CAD build for the part. Positions are in the model's coordinates, mm. Face numbers are marked on the shaded views. A direction names the side the tool comes from. Coordinates: 2 decimals unless noted, no trailing zeros. Loops run counter-clockwise (first coordinate to the right, second up) from the corner with the lowest first, then second, coordinate; pieces in that order, holes last. Notation, with made-up numbers: (-40, 86.25) -> (0, 86.25) arc R13 cw to (0, 97.25) -> close; hole circle Ø4 at (-23, 4). An arc over 180 degrees is marked (long way). Write each question's results on one line, items separated by ' | '.
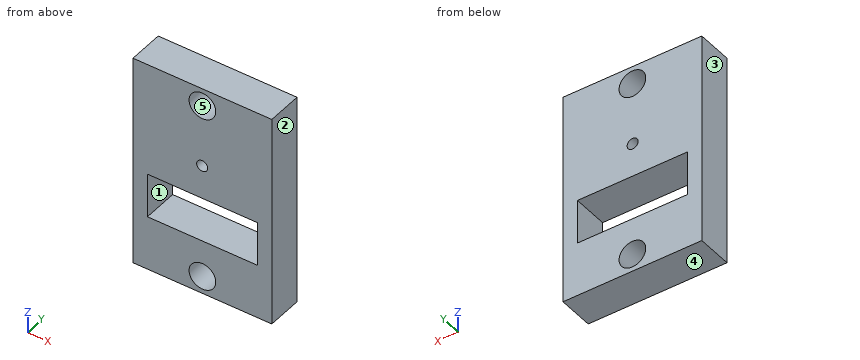
```python
from build123d import *

# Parameters (mm, degrees)
SKETCH1_W           = 78
SKETCH1_H           = 120
BOSS_EXTRUDE1_DEPTH = 10
CUT_EXTRUDE1_REACH  = 102.419
SKETCH2_W           = 61.75
SKETCH2_H           = 25
CUT_EXTRUDE2_REACH  = 102.419
SKETCH3_R           = 7.5
CUT_EXTRUDE3_REACH  = 102.419
SKETCH5_R           = 3.1


with BuildPart() as part:
    # Sketch1 → Boss-Extrude1 (new, symmetric)
    with BuildSketch(Plane(origin=(0, 0, 0), x_dir=(1, 0, 0), z_dir=(0, 1, 0))):
        with Locations((-39, 0)):
            Rectangle(SKETCH1_W, SKETCH1_H)
    extrude(amount=BOSS_EXTRUDE1_DEPTH, both=True)

    # Sketch2 → Cut-Extrude1 (cut, up to next)
    with BuildSketch(Plane(origin=(0, 10, 0), x_dir=(1, 0, 0), z_dir=(0, 1, 0)), mode=Mode.PRIVATE) as cut_extrude1_sk1:
        with Locations((-39, 16.78)):
            Rectangle(SKETCH2_W, SKETCH2_H)
    cut_extrude1_tool1 = extrude(cut_extrude1_sk1.sketch, amount=-CUT_EXTRUDE1_REACH, mode=Mode.PRIVATE) & part.part
    add(cut_extrude1_tool1.solids().sort_by_distance((-39, 10, -16.78))[0], mode=Mode.SUBTRACT)

    # Sketch3 → Cut-Extrude2 (cut, up to next)
    with BuildSketch(Plane(origin=(0, 10, 0), x_dir=(1, 0, 0), z_dir=(0, 1, 0)), mode=Mode.PRIVATE) as cut_extrude2_sk1:
        with Locations(Location((-39, 50, 0), (0, 0, 270))):
            Circle(SKETCH3_R)
    cut_extrude2_tool1 = extrude(cut_extrude2_sk1.sketch, amount=-CUT_EXTRUDE2_REACH, mode=Mode.PRIVATE) & part.part
    # Sketch3 → Cut-Extrude2 (cut, up to next)
    with BuildSketch(Plane(origin=(0, 10, 0), x_dir=(1, 0, 0), z_dir=(0, 1, 0)), mode=Mode.PRIVATE) as cut_extrude2_sk2:
        with Locations(Location((-39, -50, 0), (0, 0, 270))):
            Circle(SKETCH3_R)
    cut_extrude2_tool2 = extrude(cut_extrude2_sk2.sketch, amount=-CUT_EXTRUDE2_REACH, mode=Mode.PRIVATE) & part.part
    add(cut_extrude2_tool1.solids().sort_by_distance((-39, 10, -50))[0], mode=Mode.SUBTRACT)
    add(cut_extrude2_tool2.solids().sort_by_distance((-39, 10, 50))[0], mode=Mode.SUBTRACT)

    # Sketch5 → Cut-Extrude3 (cut, up to next)
    with BuildSketch(Plane(origin=(0, 10, 0), x_dir=(1, 0, 0), z_dir=(0, 1, 0)), mode=Mode.PRIVATE) as cut_extrude3_sk1:
        with Locations(Location((-39.125, -14.72, 0), (0, 0, 270))):
            Circle(SKETCH5_R)
    cut_extrude3_tool1 = extrude(cut_extrude3_sk1.sketch, amount=-CUT_EXTRUDE3_REACH, mode=Mode.PRIVATE) & part.part
    add(cut_extrude3_tool1.solids().sort_by_distance((-39.125, 10, 14.72))[0], mode=Mode.SUBTRACT)


solid = part.part
```
Q1. Drop a flat-ended pin along its axis: pin 1 (12 mm diameter, centred on x = -39, z = -50, fed in from +Y) (1 decimal). Give the stop position or say it passes through.
Results are:
pin 1: through
Q2. Which spindle directions (+Z, -Z, +X, -X, +Y, -Y) get a long thin tool onto all of the face, cutting with end or side? Do the marked faces 1 and 2. Say none if no direction does.
Results are:
face 1: +Y, -Y | face 2: +Z, -Z, +X, +Y, -Y
Q3. Cut at C-C on y = -2.5. Write the cut outline in (x, z) (3 decimals), and give its area (3 significant figures).
Results are:
outline: (-78, -60) -> (0, -60) -> (0, 60) -> (-78, 60) -> close; hole (-69.875, -29.28) -> (-8.125, -29.28) -> (-8.125, -4.28) -> (-69.875, -4.28) -> close; hole circle Ø15 at (-39, -50); hole circle Ø15 at (-39, 50); hole circle Ø6.2 at (-39.125, 14.72) | area: 7,430 mm^2
Q4. Cut at B-B on x = -49.5. Write the cut outline in (y, z), and give its area (3 significant figures).
Results are:
outline: (-10, -60) -> (10, -60) -> (10, -29.28) -> (-10, -29.28) -> close; (-10, -4.28) -> (10, -4.28) -> (10, 60) -> (-10, 60) -> close | area: 1,900 mm^2
Q5. Wall check: L1, parallel to X at y = -4.25, z = -50.5; L2, parallel to Z at x = -22, y = -1; L3, parallel to X at y = -1, z = 14.72 (3 decimals). Give the ranges that are in metal, low to high. Write a range as from..to.
Results are:
L1: -78..-46.48, -31.52..0 | L2: -60..-29.28, -4.28..60 | L3: -78..-42.225, -36.025..0
Q6. Cut at A-A on z = 14.72. Write the cut outline in (x, y) (3 decimals).
Results are:
outline: (-78, -10) -> (-42.225, -10) -> (-42.225, 10) -> (-78, 10) -> close; (-36.025, -10) -> (0, -10) -> (0, 10) -> (-36.025, 10) -> close
Q7. Pull direction X, two halves, no side cores. Call the marked faces 3, 4 and 5: +X half, -X half, draft (parallel to the pull), parting line (faces both ways), or undercut.
Results are:
face 3: -X half | face 4: draft | face 5: undercut
